from build123d import *

# Parameters (mm, degrees)
SKETCH_1_W          = 20
SKETCH_1_H          = 32
SKETCH_1_R          = 2.75
EXTRUDE_1_DEPTH     = 4
SKETCH_2_W          = 20
SKETCH_2_H          = 10
EXTRUDE_2_DEPTH     = 13
SKETCH_4_R          = 6.2
EXTRUDE_3_DEPTH     = 10
SKETCH_5_R          = 4.2
CUT_EXTRUDE_1_DEPTH = 13
CHAMFER_1_SIZE      = 2
SKETCH_6_R          = 5
CUT_EXTRUDE_2_DEPTH = 2


with BuildPart() as part:
    # 草图1 → 凸台-拉伸1 (new body)
    with BuildSketch(Plane.XY):
        with Locations((10, -16)):
            Rectangle(SKETCH_1_W, SKETCH_1_H)
        with Locations((10, -4)):
            Circle(SKETCH_1_R, mode=Mode.SUBTRACT)
        with Locations((10, -28)):
            Circle(SKETCH_1_R, mode=Mode.SUBTRACT)
    extrude(amount=EXTRUDE_1_DEPTH)

    # 草图2 → 凸台-拉伸2 (add)
    with BuildSketch(Plane.XY.offset(4)):
        with Locations((10, -16)):
            Rectangle(SKETCH_2_W, SKETCH_2_H)
    extrude(amount=EXTRUDE_2_DEPTH)

    # 草图4 → 凸台-拉伸3 (add)
    with BuildSketch(Plane.XZ.offset(21)):
        with Locations((10, 17)):
            Circle(SKETCH_4_R)
    extrude(amount=-EXTRUDE_3_DEPTH)

    # 草图5 → 切除-拉伸1 (cut)
    with BuildSketch(Plane(origin=(0, -11, 0), x_dir=(1, 0, 0), z_dir=(0, 1, 0))):
        with Locations(Location((10, -17, 0), (0, 0, 270))):
            Circle(SKETCH_5_R)
    extrude(amount=-CUT_EXTRUDE_1_DEPTH, mode=Mode.SUBTRACT)

    # 倒角1
    chamfer_1_edges = [part.edges().sort_by_distance(p)[0] for p in [
        (0, -11, 10.5),
        (0, -21, 10.5),
        (20, -21, 10.5),
        (20, -11, 10.5),
    ]]
    chamfer(chamfer_1_edges, length=CHAMFER_1_SIZE)

    # 草图6 → 切除-拉伸2 (cut)
    with BuildSketch(Plane.XY.offset(4)):
        with Locations((10, -28)):
            Circle(SKETCH_6_R)
        with Locations((10, -4)):
            Circle(SKETCH_6_R)
    extrude(amount=-CUT_EXTRUDE_2_DEPTH, mode=Mode.SUBTRACT)


solid = part.part
Geometry check sheet. Reference: the model listing, model coordinates, mm. A direction names the side the tool comes from. Round coordinates to 2 decimals unless told otherwise and drop trailing zeros. Order: outer loops, then holes, each group sorted by start corner. A loop starts at its lowest first (then second) coordinate and runs counter-clockwise, first axis right, second up. Notation, with made-up numbers: M -38,31 L 2,31 A26 cw 2,47 Z; hole C -25.5,-14 d10. An arc over 180 degrees is marked long. Answer in a Markdown table with one row per item. Add a question column.
Item 1: Sectioned sample at D-D, the plane z = 19. Enter the section's corners in (x, y).
Item 2: Set-up check for faces 1 (the face through (2, -16, 17)), 2 (the face through (18, -16, 17)), 3 (the face through (9, -1, 2)): record each of +Z, -Z, +X, -X, +Y, -Y from which the full face is reachable in a straight line by a thin tool's end or side.
Item 3: Sectioned sample at B-B, the plane y = -4. Enter the section's corners in (x, z), plus the area to 3 significant figures.
Item 4: Material ranges on L1, parallel to Y at x = 10, z = 1.05; L2, parallel to X at y = -28, z = 3.3; L3, parallel to Y at x = 16.5, z = 9.75, recorded low to high. Write a range as [from, to].
Item 5: Depth check by flat-ended pin: pin 1 Ø3 at (y, z) = (-8.5, 14) entering from -X; pin 2 Ø7 at (x, y) = (10, -4) entering from -Z; pin 3 Ø1.1 at (x, y) = (19, -17.5) entering from +Z; pin 4 Ø12 at (x, z) = (7.5, 15.5) entering from +Y. Enter the tip coordinate at first touch or a pass-through.
Item 6: Sectioned sample at A-A, the plane x = 10. Enter the section's corners in (y, z), plus the area to 3 significant figures.
Item 7: Sectioned sample at C-C, the plane y = -20. Enter the section's corners in (x, z).
Item 8: Draft check along Y on faces 4 (the face through (10, -21, 12)), 5 (the face through (9.9, -22.5, 4)), 6 (the face through (19, -12, 10)), 7 (the face through (9, -25, 2)). Enter one of: released by +Y, released by -Y, zero draft, split by the parting line, or undercut.
Filled in:
| question | item | result |
|---|---|---|
| 1 | outline | M 4.13,-21 L 6.31,-21 L 6.31,-11 L 4.13,-11 Z; M 13.69,-21 L 15.87,-21 L 15.87,-11 L 13.69,-11 Z |
| 2 | face 1 | +Z, -X, +Y, -Y |
| 2 | face 2 | +Z, +X, +Y, -Y |
| 2 | face 3 | +Z |
| 3 | outline | M 0,0 L 7.25,0 L 7.25,2 L 5,2 L 5,4 L 0,4 Z; M 12.75,0 L 20,0 L 20,4 L 15,4 L 15,2 L 12.75,2 Z |
| 3 | area | 49.0 mm² |
| 4 | L1 | y = [-32, -30.75], [-25.25, -6.75], [-1.25, 0] |
| 4 | L2 | x = [0, 5], [15, 20] |
| 4 | L3 | y = [-21, -11] |
| 5 | pin 1 | passes through |
| 5 | pin 2 | stops at z = 0 |
| 5 | pin 3 | stops at z = 17 |
| 5 | pin 4 | stops at y = -11 |
| 6 | outline | M -32,0 L -30.75,0 L -30.75,2 L -32,2 Z; M -25.25,0 L -6.75,0 L -6.75,2 L -9,2 L -9,4 L -11,4 L -11,12.8 L -21,12.8 L -21,4 L -23,4 L -23,2 L -25.25,2 Z; M -21,21.2 L -11,21.2 L -11,23.2 L -21,23.2 Z; M -1.25,0 L 0,0 L 0,2 L -1.25,2 Z |
| 6 | area | 178 mm² |
| 7 | outline | M 0,0 L 20,0 L 20,4 L 19,4 L 19,17 L 16.2,17 A6.2 ccw 3.8,17 L 1,17 L 1,4 L 0,4 Z; hole C 10,17 d8.4 |
| 8 | face 4 | released by -Y |
| 8 | face 5 | zero draft |
| 8 | face 6 | released by +Y |
| 8 | face 7 | undercut |
